from build123d import *

# Parameters (mm, degrees)
SKETCH1_R           = 12.7
BOSS_EXTRUDE1_DEPTH = 101.6


with BuildPart() as part:
    # Sketch1 → Boss-Extrude1 (new body)
    with BuildSketch(Plane(origin=(0, 0, 0), x_dir=(1, 0, 0), z_dir=(0, 1, 0))):
        with Locations(Location((0, 0, 0), (0, 0, 270))):
            Circle(SKETCH1_R)
    extrude(amount=BOSS_EXTRUDE1_DEPTH)

    # Sketch2 → Cut-Revolve1 (revolve, cut)
    with BuildSketch(Plane(origin=(0, 101.6, 0), x_dir=(1, 0, 0), z_dir=(0, 1, 0))):
        with BuildLine():
            Line((0, 12.7), (0, -12.7))
            ThreePointArc((0, -12.7), (12.7, 0), (0, 12.7))
        make_face()
    revolve(axis=Axis((0, 101.6, -12.7), (0, 0, 1)), mode=Mode.SUBTRACT)

    # Sketch3 → Cut-Revolve2 (revolve, cut)
    with BuildSketch(Plane(origin=(0, 0, 0), x_dir=(-1, 0, 0), z_dir=(0, -1, 0))):
        with BuildLine():
            Line((0, -10.16), (0, 10.16))
            ThreePointArc((0, 10.16), (-10.16, 0), (0, -10.16))
        make_face()
    revolve(axis=Axis((0, 0, 10.16), (0, 0, -1)), mode=Mode.SUBTRACT)


solid = part.part
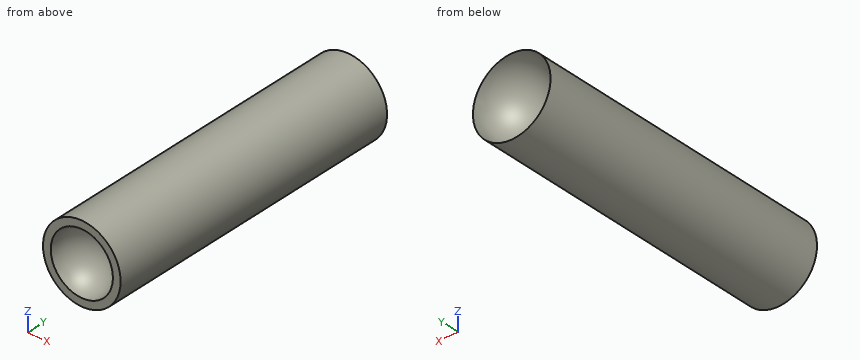
Read the model definition and answer for the solid it produces. Units are mm, in the model's axes. Give positions to 0.01 mm unless a question says otherwise; leave off trailing zeros. Write each loop counter-clockwise with the first axis right and the second up, starting at its lowest first coordinate (ties: lowest second). Pieces come first, ordered by that corner, then holes. Notation, with made-up numbers: M -13.5,24 L 23.5,24 A22 cw 23.5,53 Z; hole C -8,58.25 d3. An arc over 180 degrees is marked long. One line per item, written item: value. Start each with the question number.
(1) Find section B-B (x = 0). Determine the outline of the cut face in (y, z).
(2) Find section D-D (y = 8). Determine the outline of the cut face in (x, z), plus the area to 3 significant figures.
(3) Find section C-C (y = 49.5). Determine the outline of the cut face in (x, z).
(4) Flat-ended cylindrical pins translate along their axes: pin 1 Ø1.5 at (x, y) = (-10, 32) entering from -Z; pin 2 Ø1.5 at (x, y) = (4, 27.5) entering from +Z; pin 3 Ø8 at (x, y) = (10, 76.5) entering from -Z. Find the tip coordinate at first contact, or state that the pin passes through.
(5) Find section A-A (z = 0). Determine the outline of the cut face in (x, y).
(6) Find the intervals of material crossed by line 1 (Z direction, x = 0.75, y = 93.5); line 2 (X direction, y = 51, z = -1.75); line 3 (X direction, y = 37, z = 4), in increasing order.
Results below:
1. outline: M 0,-12.7 L 101.6,-12.7 A12.7 cw 101.6,12.7 L 0,12.7 L 0,10.16 A10.16 cw 0,-10.16 Z
2. outline: C 0,0 d25.4; hole C 0,0 d12.53
2. area: 383 mm^2
3. outline: C 0,0 d25.4
4. pin 1: stops at z = -8.7
4. pin 2: stops at z = 12.28
4. pin 3: stops at z = -11.19
5. outline: M -12.7,0 L -10.16,0 A10.16 cw 10.16,0 L 12.7,0 L 12.7,101.6 A12.7 cw -12.7,101.6 Z
6. line 1: z = -12.68 to -9.75, 9.75 to 12.68
6. line 2: x = -12.58 to 12.58
6. line 3: x = -12.05 to 12.05
